from build123d import *

# Parameters (mm, degrees)
BOSS_EXTRUDE2_DEPTH                                 = 4
CSK_FOR_M3_COUNTERSUNK_FLAT_HEAD_SCREW1_D           = 3.4
CSK_FOR_M3_COUNTERSUNK_FLAT_HEAD_SCREW1_CSINK_D     = 6.3
CSK_FOR_M3_COUNTERSUNK_FLAT_HEAD_SCREW1_CSINK_ANGLE = 90
CUT_EXTRUDE1_REACH                                  = 103.316
SKETCH5_R                                           = 25
CUT_EXTRUDE2_DEPTH                                  = 1
CHAMFER3_SIZE                                       = 3.99


with BuildPart() as part:
    # Sketch1 → Boss-Extrude2 (new body)
    with BuildSketch(Plane.XY):
        with BuildLine():
            Line((-33.226495452, -67.238381896), (33.226495452, -67.238381896))
            ThreePointArc((33.226495452, -67.238381896), (74.994830614, 0.880557322), (31.638584039, 68))
            Line((31.638584039, 68), (-31.638584039, 68))
            ThreePointArc((-31.638584039, 68), (-74.994830614, 0.880557322), (-33.226495452, -67.238381896))
        make_face()
    extrude(amount=BOSS_EXTRUDE2_DEPTH)

    # CSK for M3 Countersunk Flat Head Screw1 (through all)
    with Locations(Plane.XY.offset(4)):
        with Locations((-15, -37.238381896), (0, -51.238381896), (15, -37.238381896)):
            CounterSinkHole(CSK_FOR_M3_COUNTERSUNK_FLAT_HEAD_SCREW1_D / 2, CSK_FOR_M3_COUNTERSUNK_FLAT_HEAD_SCREW1_CSINK_D / 2, counter_sink_angle=CSK_FOR_M3_COUNTERSUNK_FLAT_HEAD_SCREW1_CSINK_ANGLE)

    # Sketch4 → Cut-Extrude1 (cut, up to next)
    with BuildSketch(Plane.XY.offset(4), mode=Mode.PRIVATE) as cut_extrude1_sk1:
        with BuildLine():
            Line((-8, 16), (-8, 68))
            Line((-8, 68), (8, 68))
            Line((8, 68), (8, 16))
            ThreePointArc((8, 16), (0, 8), (-8, 16))
        make_face()
    cut_extrude1_tool1 = extrude(cut_extrude1_sk1.sketch, amount=-CUT_EXTRUDE1_REACH, mode=Mode.PRIVATE) & part.part
    add(cut_extrude1_tool1.solids().sort_by_distance((0, 38.831056, 4))[0], mode=Mode.SUBTRACT)

    # Sketch5 → Cut-Extrude2 (cut)
    with BuildSketch(Plane.XY.offset(4)):
        with Locations((0, 61.9)):
            Circle(SKETCH5_R)
    extrude(amount=-CUT_EXTRUDE2_DEPTH, mode=Mode.SUBTRACT)

    # Chamfer3
    chamfer3_edges = [part.edges().sort_by_distance(p)[0] for p in [
        (74.994830614, 0.880557322, 0),
        (-74.994830614, 0.880557322, 0),
    ]]
    chamfer(chamfer3_edges, length=CHAMFER3_SIZE)


solid = part.part
The model under review builds one solid part; all positions refer to its coordinate system, in mm. A direction names the side the tool comes from. Coordinates: 2 decimals unless noted, no trailing zeros. Loops run counter-clockwise (first coordinate to the right, second up) from the corner with the lowest first, then second, coordinate; pieces in that order, holes last. Notation, with made-up numbers: M 56,25 L 115,25 A32 cw 115,59 Z; hole C -5.5,79.25 d3. An arc over 180 degrees is marked long. Put each result on its own line as item: value. Start each with the question number.
Q1. The part is to be moulded in two halves that separate along X. For faces 3 (the cylindrical face through (14.22, -38.75, 1.26)), 4 (the flat face through (0, -67.238, 2)), 5 (the conical face through (71.26, 0, 0.25)), say which applies: +X half, -X half, draft (parallel to the pull), parting line (faces both ways), or undercut.
Q2. Wall thickness on line 1 (Y direction, x = -15, z = 1.45); line 2 (Y direction, x = 0, z = 0.8); line 3 (X direction, y = 20, z = 0.5): over which ranges is each line inside the solid? List them lowest first.
Q3. Add section A-A (x = -15). Write out the cut boundary in (y, z).
Q4. For faces 1 (the flat face through (-8, 42, 2)), 2 (the cylindrical face through (-16.57, -37.89, 1.26)), list the 3-axis set-ups (+Z, -Z, +X, -X, +Y, -Y) from which the entire face can be reached by the end or side of a thin tool; tool diameter is ignored.
Q5. Clearance check with flat-ended pins moving along their axes: pin 1 (13.5 mm diameter, centred on x = -16, y = 54, fed in from +Z); pin 2 (2 mm diameter, centred on y = -52.5, z = 1.5, fed in from -X); pin 3 (1.2 mm diameter, centred on y = 51, z = 2, fed in from +X). State where each tip first meets the part, or that it passes through.
Q6. Add section B-B (z = 1). Write out the cut boundary in (x, y).
Answers:
1. face 3: undercut
1. face 4: draft
1. face 5: +X half
2. line 1: y = -67.24 to -38.94, -35.54 to 68
2. line 2: y = -67.24 to -52.94, -49.54 to 8
2. line 3: x = -68.66 to -8, 8 to 68.66
3. outline: M -67.24,0 L -38.94,0 L -38.94,2.55 L -40.39,4 L -67.24,4 Z; M -35.54,0 L 68,0 L 68,3 L 41.9,3 L 41.9,4 L -34.09,4 L -35.54,2.55 Z
4. face 1: +Z, -Z, +Y
4. face 2: +Z, -Z
5. pin 1: stops at z = 3
5. pin 2: stops at x = -51.78
5. pin 3: stops at x = 53.26
6. outline: M -25.78,-67.24 L 25.78,-67.24 A72.01 ccw 23.69,68 L 8,68 L 8,16 A8 cw -8,16 L -8,68 L -23.69,68 A72.01 ccw Z; hole C -15,-37.24 d3.4; hole C 0,-51.24 d3.4; hole C 15,-37.24 d3.4
